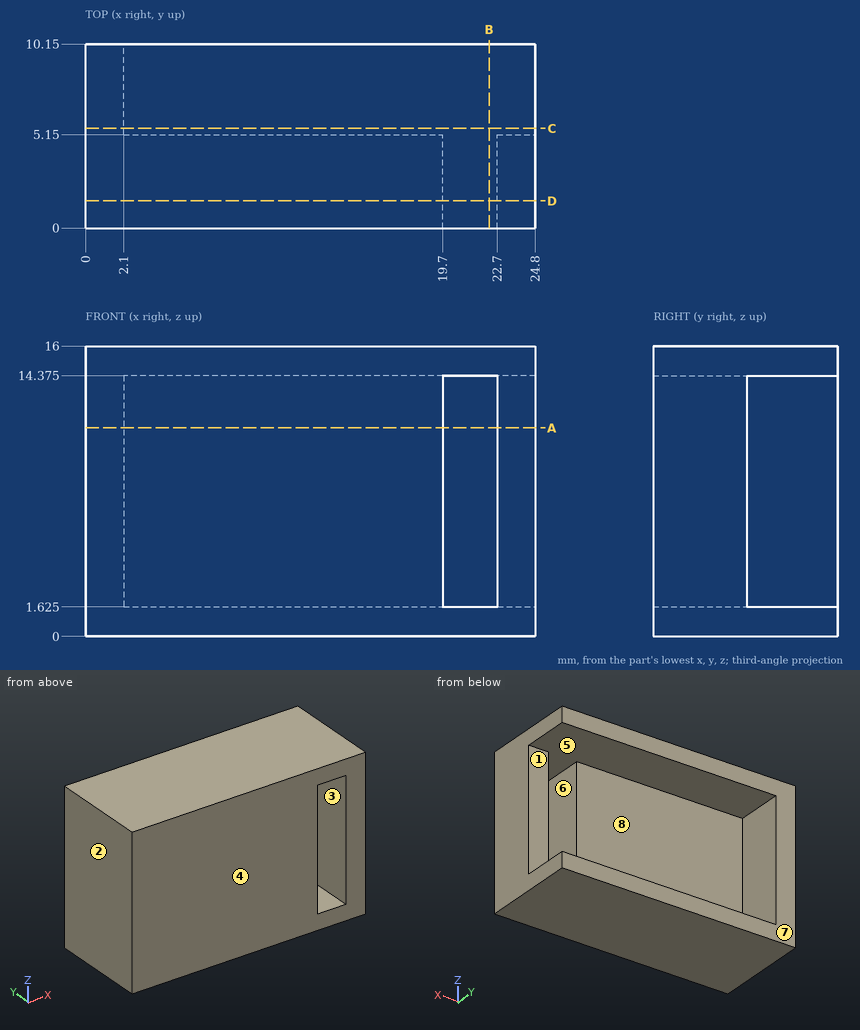
Verification items for this drawing (mm, ordinates from the low corner). A direction names the side the tool comes from. Coordinates: 2 decimals unless noted, no trailing zeros. Order: outer loops, then holes, each group sorted by start corner. A loop starts at its lowest first (then second) coordinate and runs counter-clockwise, first axis right, second up.
Q1. Draft check along X on the marked faces 1, 2 and 3. Enter one of: released by +X, released by -X, zero draft, split by the parting line, or undercut.
Reply:
face 1: zero draft
face 2: released by -X
face 3: undercut
Q2. Sectioned sample at A-A on z = 11.5. Record the cut outline in (x, y), and give its area (3 significant figures).
Reply:
outline: (0, 0) - (19.7, 0) - (19.7, 5.15) - (2.1, 5.15) - (2.1, 10.15) - (0, 10.15) - close; (22.7, 0) - (24.8, 0) - (24.8, 5.15) - (22.7, 5.15) - close
area: 123 mm2
Q3. Sectioned sample at D-D on y = 1.5. Record the cut outline in (x, z) (3 decimals).
Reply:
outline: (0, 0) - (24.8, 0) - (24.8, 16) - (0, 16) - close; hole (19.7, 1.625) - (22.7, 1.625) - (22.7, 14.375) - (19.7, 14.375) - close
Q4. Sectioned sample at C-C on y = 5.5. Record the cut outline in (x, z) (3 decimals), and give its area (3 significant figures).
Reply:
outline: (0, 0) - (24.8, 0) - (24.8, 1.625) - (2.1, 1.625) - (2.1, 14.375) - (24.8, 14.375) - (24.8, 16) - (0, 16) - close
area: 107 mm2
Q5. Depth check by flat-ended pin: pin 1 Ø0.6 at (x, z) = (24, 8.5) entering from +Y; pin 2 Ø1.5 at (y, z) = (8, 8.5) entering from +X. Enter the tip coordinate at first touch or a pass-through.
Reply:
pin 1: stops at y = 5.15
pin 2: stops at x = 2.1
Q6. Sectioned sample at B-B on x = 22.25. Record the cut outline in (y, z) (3 decimals), and give its area (3 significant figures).
Reply:
outline: (0, 0) - (10.15, 0) - (10.15, 1.625) - (0, 1.625) - close; (0, 14.375) - (10.15, 14.375) - (10.15, 16) - (0, 16) - close
area: 33.0 mm2
Q7. Tool access check on the marked faces 4, 5, 6, 7 and 8. Record the directions out of +Z, -Z, +X, -X, +Y, -Y that give a thin tool (end or side, any length) a straight path to the whole face; none if there is none.
Reply:
face 4: +Z, -Z, +X, -X, -Y
face 5: +Y
face 6: +Y, -Y
face 7: +Z, -Z, +X, -X, +Y
face 8: +X, +Y
Q8. Thickness scan on probe 1 along X at (y, z) = (1.5, 9.75); probe 2 along Z at (x, y) = (22.25, 7.5) (3 decimals); probe 3 along Y at (x, z) = (6.5, 13.5). Record the ranges inside material, lowest first.
Reply:
probe 1: x = 0 to 19.7, 22.7 to 24.8
probe 2: z = 0 to 1.625, 14.375 to 16
probe 3: y = 0 to 5.15
